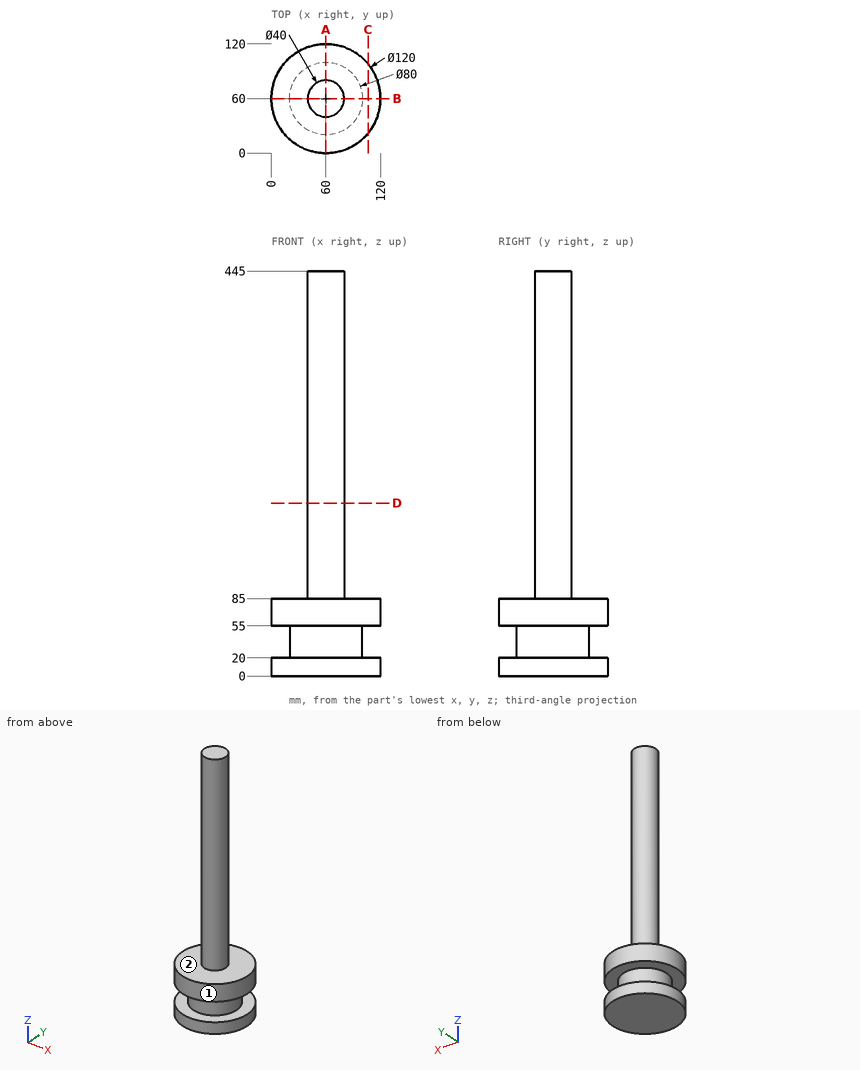
For this review, use the dimensioned drawing (mm, ordinates from the lowest corner) and the shaded views. A direction names the side the tool comes from. Coordinates: 2 decimals unless noted, no trailing zeros. Loops run counter-clockwise (first coordinate to the right, second up) from the corner with the lowest first, then second, coordinate; pieces in that order, holes last.
1. For the marked faces 1 and 2, list the 3-axis set-ups (+Z, -Z, +X, -X, +Y, -Y) from which the entire face can be reached by the end or side of a thin tool; tool diameter is ignored.
2. Add section D-D, the plane z = 190. Give the boundary of the cut face in (x, y), then the cut area to 3 significant figures.
3. Add section C-C, the plane x = 106.5. Give the boundary of the cut face in (y, z).
4. Add section A-A, the plane x = 60. Give the boundary of the cut face in (y, z).
5. Insertion check: P1, Ø6, axis at y = 63.5, z = 209, coming from the +X side; P2, Ø1, axis at x = 76, y = 81, coming from the +Z side; P3, Ø12, axis at x = 52, z = 287.5, coming from the +Y side. Each pin has a flat end and moves straight along its axis. Give the tip position at first contact, or say it passes through.
6. For line 1 (Z direction, x = 79, y = 103); line 2 (Z direction, x = 58, y = 35.5); line 3 (X direction, y = 60, z = 237), list the stretches that pass through material, from the lowest coordinate up.
Result:
1. face 1: +Z, -Z
1. face 2: +Z
2. outline: circle Ø40 at (60, 60)
2. area: 1,260 mm2
3. outline: (22.08, 0) - (97.92, 0) - (97.92, 20) - (22.08, 20) - close; (22.08, 55) - (97.92, 55) - (97.92, 85) - (22.08, 85) - close
4. outline: (0, 0) - (120, 0) - (120, 20) - (100, 20) - (100, 55) - (120, 55) - (120, 85) - (80, 85) - (80, 445) - (40, 445) - (40, 85) - (0, 85) - (0, 55) - (20, 55) - (20, 20) - (0, 20) - close
5. P1: stops at x = 79.99
5. P2: stops at z = 85
5. P3: stops at y = 79.9
6. line 1: z = 0 to 20, 55 to 85
6. line 2: z = 0 to 85
6. line 3: x = 40 to 80
